Input: part model. Units: mm. Frame: model coordinates. Face numbers are marked on the shaded views. A direction names the side the tool comes from. Round coordinates to 2 decimals unless told otherwise and drop trailing zeros. Order: outer loops, then holes, each group sorted by start corner. A loop starts at its lowest first (then second) coordinate and runs counter-clockwise, first axis right, second up. Notation, with made-up numbers: (18.5, 56.25) -> (60.5, 56.25) arc R18 ccw to (60.5, 72.25) -> close; hole circle Ø3 at (58.25, -3). An arc over 180 degrees is marked (long way). Use a Markdown table: item, result.
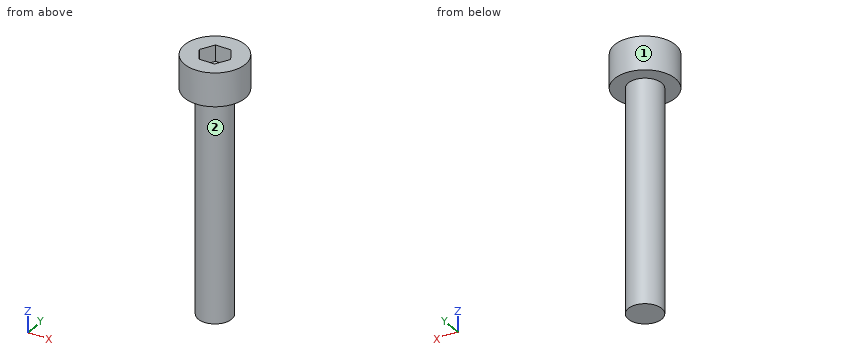
from build123d import *

# Parameters (mm, degrees)
SKETCH1_W           = 2.725
SKETCH1_H           = 3
SKETCH2_R           = 1.5
BOSS_EXTRUDE1_DEPTH = 3
SKETCH3_R           = 1.5
BOSS_EXTRUDE2_DEPTH = 17
CUT_EXTRUDE1_DEPTH  = 1.45


with BuildPart() as part:
    # Sketch1 → Revolve1 (revolve)
    with BuildSketch(Plane(origin=(0, 0, 0), x_dir=(1, 0, 0), z_dir=(0, 1, 0))):
        with Locations((1.3625, 1.5)):
            Rectangle(SKETCH1_W, SKETCH1_H)
    revolve(axis=Axis((0, 0, -3), (0, 0, 1)))

    # Sketch2 → Boss-Extrude1 (add)
    with BuildSketch(Plane(origin=(0, 0, -3), x_dir=(-1, 0, 0), z_dir=(0, 0, -1))):
        Circle(SKETCH2_R)
    extrude(amount=BOSS_EXTRUDE1_DEPTH)

    # Sketch3 → Boss-Extrude2 (add)
    with BuildSketch(Plane(origin=(0, 0, -6), x_dir=(-1, 0, 0), z_dir=(0, 0, -1))):
        Circle(SKETCH3_R)
    extrude(amount=BOSS_EXTRUDE2_DEPTH)

    # Sketch4 → Cut-Extrude1 (cut)
    with BuildSketch(Plane.XY):
        Polygon((-1.4, 0), (-0.7, -1.212435565), (0.7, -1.212435565), (1.4, 0), (0.7, 1.212435565), (-0.7, 1.212435565), align=None)
    extrude(amount=-CUT_EXTRUDE1_DEPTH, mode=Mode.SUBTRACT)


solid = part.part
1) Pin query (flat end, axial travel): pin 1 Ø1.5 at (x, y) = (-1.5, 2) entering from -Z; pin 2 Ø3 at (x, z) = (-1.5, -18) entering from -Y; pin 3 Ø1.5 at (x, z) = (-1, -7.5) entering from +Y; pin 4 Ø2.5 at (x, y) = (0.5, 0) entering from +Z. Return the tip coordinate at first contact, or that it passes through.
Results found:
| item | result |
|---|---|
| pin 1 | stops at z = -3 |
| pin 2 | stops at y = -1.5 |
| pin 3 | stops at y = 1.48 |
| pin 4 | stops at z = 0 |
2) Cut plane A-A on x = 0. Return loops of the section in (y, z) (3 decimals), and give its area (3 significant figures).
Results found:
| item | result |
|---|---|
| outline | (-2.725, -3) -> (-1.5, -3) -> (-1.5, -23) -> (1.5, -23) -> (1.5, -3) -> (2.725, -3) -> (2.725, 0) -> (1.212, 0) -> (1.212, -1.45) -> (-1.212, -1.45) -> (-1.212, 0) -> (-2.725, 0) -> close |
| area | 72.8 mm² |
3) Cut plane D-D on x = 1.85. Return loops of the section in (y, z).
Results found:
| item | result |
|---|---|
| outline | (-2, -3) -> (2, -3) -> (2, 0) -> (-2, 0) -> close |
4) Cut plane C-C on z = -16.25. Return loops of the section in (x, y), and give its area (3 significant figures).
Results found:
| item | result |
|---|---|
| outline | circle Ø3 at (0, 0) |
| area | 7.07 mm² |
5) Line query: L1, parallel to Z at x = 2.1, y = 0.65; L2, parallel to Z at x = -0.9, y = 0.25; L3, parallel to Y at x = 0, z = -21. Output: solid intervals per line, ascending. Write a range as [from, to].
Results found:
| item | result |
|---|---|
| L1 | z = [-3, 0] |
| L2 | z = [-23, -1.45] |
| L3 | y = [-1.5, 1.5] |
6) Set-up query: the marked faces 1 and 2. Return all of +Z, -Z, +X, -X, +Y, -Y with unobstructed straight access to the full face (end or side cutting, diameter ignored); none if empty.
Results found:
| item | result |
|---|---|
| face 1 | +Z, -Z |
| face 2 | -Z |
7) Cut plane B-B on y = 0.9. Return loops of the section in (x, z), and give its area (3 significant figures).
Results found:
| item | result |
|---|---|
| outline | (-2.57, -3) -> (-1.2, -3) -> (-1.2, -23) -> (1.2, -23) -> (1.2, -3) -> (2.57, -3) -> (2.57, 0) -> (0.88, 0) -> (0.88, -1.45) -> (-0.88, -1.45) -> (-0.88, 0) -> (-2.57, 0) -> close |
| area | 60.9 mm² |
